Source: CAD feature listing. Evaluate the final solid. Frame: model axes, mm. A direction names the side the tool comes from. Round coordinates to 2 decimals unless told otherwise and drop trailing zeros. Order: outer loops, then holes, each group sorted by start corner. A loop starts at its lowest first (then second) coordinate and runs counter-clockwise, first axis right, second up. Notation, with made-up numbers: (63.5, 13.5) - (75.5, 13.5) arc R26 cw to (75.5, 36.5) - close; hole circle Ø11 at (-40, -26.5). An arc over 180 degrees is marked (long way). Return JSON: item names as keys, results as strings. Group by question number.
1) Ray query, line 1 (Z direction, x = 2.25, y = 0); line 2 (Y direction, x = 2, z = 6.25); line 3 (Z direction, x = 1.85, y = -1.75). Return the intervals inside material, ascending. Write a range as from..to.
2) Access query for faces 1 (the flat face through (1, 0, -4)), 2 (the flat face through (1, 4, 4)), 3 (the flat face through (1, -4, 4)). Directions: +Z, -Z, +X, -X, +Y, -Y. A direction counts if a zero-diameter tool reaches every point of the face in a straight line with its end or side. Return the directions, or none.
3) Section C-C, the plane x = 1.2. Return loops of the section in (y, z), plus the area to 3 significant figures.
4) Section B-B, the plane z = 0. Return loops of the section in (x, y).
5) Section A-A, the plane y = 0. Return loops of the section in (x, z).
6) Section D-D, the plane z = 5.75. Return loops of the section in (x, y).
7) Contact query for flat-ended pins moving along their axis: P1, Ø1.4, axis at x = 1, y = 4.5, coming from the +Z side; P2, Ø1.5, axis at x = 1, z = 5, coming from the -Y side; P3, Ø4.5, axis at y = 0, z = 0, coming from the -X side. Output: stop coordinate, or through.
```python
from build123d import *

# Parameters (mm, degrees)
F0_R     = 2.5
F1_DEPTH = 3


with BuildPart() as f1:
    # F0 (on Right) → F1 (new body)
    with BuildSketch(Plane.YZ):
        Polygon((-5, 4), (-5, -4), (5, -4), (5, 4), (3.75, 4), (3.75, 7), (-3.75, 7), (-3.75, 4), align=None)
        Circle(F0_R, mode=Mode.SUBTRACT)
    extrude(amount=F1_DEPTH)


solid = f1.part
```
Geometry check:
{
 "1": {"line 1": "-4..-2.5, 2.5..7", "line 2": "-3.75..3.75", "line 3": "-4..-1.79, 1.79..7"},
 "2": {"face 1": "-Z, +X, -X, +Y, -Y", "face 2": "+Z, +X, -X, +Y", "face 3": "+Z, +X, -X, -Y"},
 "3": {"outline": "(-5, -4) - (5, -4) - (5, 4) - (3.75, 4) - (3.75, 7) - (-3.75, 7) - (-3.75, 4) - (-5, 4) - close; hole circle Ø5 at (0, 0)", "area": "82.9 mm2"},
 "4": {"outline": "(0, -5) - (3, -5) - (3, -2.5) - (0, -2.5) - close; (0, 2.5) - (3, 2.5) - (3, 5) - (0, 5) - close"},
 "5": {"outline": "(0, -4) - (3, -4) - (3, -2.5) - (0, -2.5) - close; (0, 2.5) - (3, 2.5) - (3, 7) - (0, 7) - close"},
 "6": {"outline": "(0, -3.75) - (3, -3.75) - (3, 3.75) - (0, 3.75) - close"},
 "7": {"P1": "z = 4", "P2": "y = -3.75", "P3": "through"}
}
